```python
from build123d import *

# Parameters (mm, degrees)
SK_MAIN_EXTRUSION_R  = 3.4
MAIN_EXTRUSION_DEPTH = 25


with BuildPart() as part:
    # Sk Main Extrusion → Main Extrusion (new body)
    with BuildSketch(Plane.XY):
        with BuildLine():
            Line((5.926823816, -15.329316686), (19, -15.329316686))
            ThreePointArc((19, -15.329316686), (19.68041035, -15.166119497), (20.212765957, -14.712039028))
            ThreePointArc((20.212765957, -14.712039028), (0, 25), (-20.212765957, -14.712039028))
            ThreePointArc((-20.212765957, -14.712039028), (-19.68041035, -15.166119497), (-19, -15.329316686))
            Line((-19, -15.329316686), (-5.926823816, -15.329316686))
            ThreePointArc((-5.926823816, -15.329316686), (-5.496641489, -15.193680719), (-5.222054351, -14.835831793))
            Line((-5.222054351, -14.835831793), (-4.190076845, -12.000496898))
            ThreePointArc((-4.190076845, -12.000496898), (-4.175951325, -11.893202927), (-4.208493649, -11.789991862))
            Line((-4.208493649, -11.789991862), (-4.987558066, -10.44061271))
            Line((-4.987558066, -10.44061271), (-5.718509166, -10.174568267))
            Line((-5.718509166, -10.174568267), (-8.396186179, -11.149162996))
            ThreePointArc((-8.396186179, -11.149162996), (-8.811074612, -11.115806485), (-9.056960151, -10.779971153))
            ThreePointArc((-9.056960151, -10.779971153), (-8.933433013, -7.995199058), (-7.504160339, -5.602001573))
            Line((-7.504160339, -5.602001573), (-6.540737726, -4.63857896))
            ThreePointArc((-6.540737726, -4.63857896), (0, -1.929316686), (6.540737726, -4.63857896))
            Line((6.540737726, -4.63857896), (7.504160339, -5.602001573))
            ThreePointArc((7.504160339, -5.602001573), (8.933433013, -7.995199058), (9.056960151, -10.779971153))
            ThreePointArc((9.056960151, -10.779971153), (8.811074612, -11.115806485), (8.396186179, -11.149162996))
            Line((8.396186179, -11.149162996), (5.718509166, -10.174568267))
            Line((5.718509166, -10.174568267), (4.987558066, -10.44061271))
            Line((4.987558066, -10.44061271), (4.208493649, -11.789991862))
            ThreePointArc((4.208493649, -11.789991862), (4.175951325, -11.893202927), (4.190076845, -12.000496898))
            Line((4.190076845, -12.000496898), (5.222054351, -14.835831793))
            ThreePointArc((5.222054351, -14.835831793), (5.496641489, -15.193680719), (5.926823816, -15.329316686))
        make_face()
        with Locations((0, 4.670683314)):
            Circle(SK_MAIN_EXTRUSION_R, mode=Mode.SUBTRACT)
        with BuildLine():
            Line((4.418969224, 0.9), (22.656787063, 0.9))
            ThreePointArc((22.656787063, 0.9), (23.021079872, 1.05752263), (23.155835236, 1.430837004))
            ThreePointArc((23.155835236, 1.430837004), (16.404877324, 16.404877324), (1.430837004, 23.155835236))
            ThreePointArc((1.430837004, 23.155835236), (1.05752263, 23.021079872), (0.9, 22.656787063))
            Line((0.9, 22.656787063), (0.9, 10.402175266))
            ThreePointArc((0.9, 10.402175266), (1.006730351, 10.093405153), (1.281355932, 9.916455609))
            ThreePointArc((1.281355932, 9.916455609), (5.109952698, 6.416645349), (4.223439612, 1.305782448))
            ThreePointArc((4.223439612, 1.305782448), (4.193751982, 1.041477219), (4.418969224, 0.9))
        make_face(mode=Mode.SUBTRACT)
        with BuildLine():
            Line((-22.656787063, 0.9), (-4.418969224, 0.9))
            ThreePointArc((-4.418969224, 0.9), (-4.193751982, 1.041477219), (-4.223439612, 1.305782448))
            ThreePointArc((-4.223439612, 1.305782448), (-5.109952698, 6.416645349), (-1.281355932, 9.916455609))
            ThreePointArc((-1.281355932, 9.916455609), (-1.006730351, 10.093405153), (-0.9, 10.402175266))
            Line((-0.9, 10.402175266), (-0.9, 22.656787063))
            ThreePointArc((-0.9, 22.656787063), (-1.05752263, 23.021079872), (-1.430837004, 23.155835236))
            ThreePointArc((-1.430837004, 23.155835236), (-16.404877324, 16.404877324), (-23.155835236, 1.430837004))
            ThreePointArc((-23.155835236, 1.430837004), (-23.021079872, 1.05752263), (-22.656787063, 0.9))
        make_face(mode=Mode.SUBTRACT)
        with BuildLine():
            Line((-18.588354061, -13.529316686), (-10.922546302, -13.529316686))
            ThreePointArc((-10.922546302, -13.529316686), (-10.501898529, -13.299604404), (-10.467762595, -12.821538488))
            ThreePointArc((-10.467762595, -12.821538488), (-11.026944485, -8.37379017), (-8.949307842, -4.401564664))
            Line((-8.949307842, -4.401564664), (-7.813529932, -3.265786754))
            ThreePointArc((-7.813529932, -3.265786754), (-6.612567589, -2.226269195), (-5.274974996, -1.369675148))
            ThreePointArc((-5.274974996, -1.369675148), (-5.152018108, -1.088432098), (-5.394318321, -0.9))
            Line((-5.394318321, -0.9), (-22.656787063, -0.9))
            ThreePointArc((-22.656787063, -0.9), (-23.021079872, -1.05752263), (-23.155835236, -1.430837004))
            ThreePointArc((-23.155835236, -1.430837004), (-21.898586855, -7.661063488), (-18.997789172, -13.31630604))
            ThreePointArc((-18.997789172, -13.31630604), (-18.819119443, -13.472878788), (-18.588354061, -13.529316686))
        make_face(mode=Mode.SUBTRACT)
        with BuildLine():
            Line((7.813529932, -3.265786754), (8.949307842, -4.401564664))
            ThreePointArc((8.949307842, -4.401564664), (11.026944485, -8.37379017), (10.467762595, -12.821538488))
            ThreePointArc((10.467762595, -12.821538488), (10.501898529, -13.299604404), (10.922546302, -13.529316686))
            Line((10.922546302, -13.529316686), (18.588354061, -13.529316686))
            ThreePointArc((18.588354061, -13.529316686), (18.819119443, -13.472878788), (18.997789172, -13.31630604))
            ThreePointArc((18.997789172, -13.31630604), (21.898586855, -7.661063488), (23.155835236, -1.430837004))
            ThreePointArc((23.155835236, -1.430837004), (23.021079872, -1.05752263), (22.656787063, -0.9))
            Line((22.656787063, -0.9), (5.394318321, -0.9))
            ThreePointArc((5.394318321, -0.9), (5.152018108, -1.088432098), (5.274974996, -1.369675148))
            ThreePointArc((5.274974996, -1.369675148), (6.612567589, -2.226269195), (7.813529932, -3.265786754))
        make_face(mode=Mode.SUBTRACT)
    extrude(amount=-MAIN_EXTRUSION_DEPTH)


solid = part.part
```
The listing builds one solid part. Answer for the finished solid, in the listing's coordinates (mm). A direction names the side the tool comes from. Coordinates: 2 decimals unless noted, no trailing zeros. Write each loop counter-clockwise with the first axis right and the second up, starting at its lowest first coordinate (ties: lowest second). Pieces come first, ordered by that corner, then holes. Notation, with made-up numbers: (-28, 16) - (-9, 16) arc R7 ccw to (-9, 22) - close; hole circle Ø4 at (79, -27). An arc over 180 degrees is marked (long way). One line per item, written item: value.
1) Find section B-B (y = 19). Give the vertices of the cut face in (x, z).
Geometry check:
outline: (-16.25, -25) - (-13.31, -25) - (-13.31, 0) - (-16.25, 0) - close; (-0.9, -25) - (0.9, -25) - (0.9, 0) - (-0.9, 0) - close; (13.31, -25) - (16.25, -25) - (16.25, 0) - (13.31, 0) - close
2) Find section C-C (x = 21). Give the vertices of the cut face in (y, z), and give its area (3 significant figures).
Geometry check:
outline: (-13.56, -25) - (-9.86, -25) - (-9.86, 0) - (-13.56, 0) - close; (-0.9, -25) - (0.9, -25) - (0.9, 0) - (-0.9, 0) - close; (9.86, -25) - (13.56, -25) - (13.56, 0) - (9.86, 0) - close
area: 230 mm2
3) Find section D-D (z = -8.75). Count the separate pieces of the cut face and the enclosed holes in it, and give its area (3 significant figures).
Geometry check:
separate pieces: 1
enclosed holes: 5
area: 488 mm2
4) Consider line 1 along Y through (x, z) = (0, -7.5); line 2 along X through (y, z) = (12.5, -21.25); line 3 along X through (y, z) = (-12, -22.75). Determine where each line is inside the solid, lowest interval first. Write a range as from..to.
Geometry check:
line 1: y = -1.93..1.27, 8.07..25
line 2: x = -21.65..-19.54, -0.9..0.9, 19.54..21.65
line 3: x = -21.93..-19.86, -10.79..-4.19, 4.19..10.79, 19.86..21.93
5) For a pull along Y with two mould halves and no side action, classify faces 1 (the cylindrical face through (19.67, -15.17, -12.32)), 2 (the cylindrical face through (-8.945, -8.033, -12.325)), 3 (the flat face through (-2, 0, -25)) as pulls with the +Y half, pulls with the -Y half, needs draft (parallel to the pull), parting line crosses it, or undercut.
Geometry check:
face 1: pulls with the -Y half
face 2: undercut
face 3: needs draft
6) A tool of negligible diameter and unlimited length cuts with its end or side. For faces 4 (the flat face through (-4.593, -11.125, -12.325)), 5 (the flat face through (-2, 0, 0)), 6 (the flat face through (-4.7, -13.4, -12.3)), from which of +Z, -Z, +X, -X, +Y, -Y can it reach the whole face along a straight path? Write none if from no direction.
Geometry check:
face 4: +Z, -Z
face 5: +Z, +X, -X, +Y, -Y
face 6: +Z, -Z, -Y
7) Find section A-A (x = 0). Give the vertices of the cut face in (y, z).
Geometry check:
outline: (-1.93, -25) - (1.27, -25) - (1.27, 0) - (-1.93, 0) - close; (8.07, -25) - (25, -25) - (25, 0) - (8.07, 0) - close
8) Each of these flat-tipped pins is pushed along its axis until it touches: pin 1 Ø8 at (y, z) = (-5, -22) entering from +X; pin 2 Ø12 at (x, z) = (-10.5, -5.5) entering from +Y; pin 3 Ø5 at (y, z) = (20.5, -4.5) entering from -X; pin 4 Ø4 at (x, y) = (0, 4.67) entering from -Z. Where does it stop, or does it pass through?
Geometry check:
pin 1: stops at x = 24.98
pin 2: stops at y = 24.59
pin 3: stops at x = -17.35
pin 4: passes through
